Input: part model. Units: mm. Frame: model coordinates. Give positions to 0.01 mm unless a question says otherwise; leave off trailing zeros. Loops run counter-clockwise (first coordinate to the right, second up) from the corner with the lowest first, then second, coordinate; pieces in that order, holes last. Notation, with made-up numbers: M 48,70 L 89,70 A12 cw 89,76 Z; hole C 50,34 d6. An arc over 180 degrees is marked long. Use CSV: the item, a comma, the result in double quotes. Start each with the question number.
Q1. Section A-A, the plane y = -4.25. Output: boundary loops of the cut face in (x, z), plus the area to 3 significant figures.
Q2. Section B-B, the plane z = 21.5. Output: boundary loops of the cut face in (x, y), plus the area to 3 significant figures.
Q3. Material intervals for line 1 along Z through (x, y) = (66, -1); line 2 along X through (y, z) = (-3.5, 13), sorted ascending.
Q4. Section C-C, the plane x = -14. Output: boundary loops of the cut face in (y, z), plus the area to 3 significant figures.
Q5. Pin query (flat end, axial travel): pin 1 (1.9 mm diameter, centred on y = -4.5, z = -3.5, fed in from -X); pin 2 (1.9 mm diameter, centred on x = -59.5, y = -2.5, fed in from -Z); pin 3 (3 mm diameter, centred on y = -4, z = 89, fed in from +X). Return the tip coordinate at first contact, or that it passes through.
from build123d import *

# Parameters (mm, degrees)
F0_W     = 152.4
F0_H     = 101.6
F1_DEPTH = 6.35
F2_W     = 25.4
F2_H     = 6.35
F3_DEPTH = 6.35
F4_W     = 6.35
F4_H     = 25.4
F5_DEPTH = 25.4


with BuildPart() as f1:
    # F0 (on Front) → F1 (new body)
    with BuildSketch(Plane.XZ):
        with Locations((0, 50.8)):
            Rectangle(F0_W, F0_H)
    extrude(amount=F1_DEPTH)

    # F2 (on face) → F3 (join)
    with BuildSketch(Plane.XZ.offset(6.35)):
        with Locations((38.1, -3.175)):
            Rectangle(F2_W, F2_H)
        with Locations((-38.1, -3.175)):
            Rectangle(F2_W, F2_H)
    extrude(amount=-F3_DEPTH)

    # F4 (on face) → F5 (cut)
    with BuildSketch(Plane.XZ.offset(6.35)):
        with Locations((73.025, 88.9)):
            Rectangle(F4_W, F4_H)
        with Locations((73.025, 12.7)):
            Rectangle(F4_W, F4_H)
        with Locations((-73.025, 12.7)):
            Rectangle(F4_W, F4_H)
        with Locations((-73.025, 88.9)):
            Rectangle(F4_W, F4_H)
    extrude(amount=-F5_DEPTH, mode=Mode.SUBTRACT)


solid = f1.part
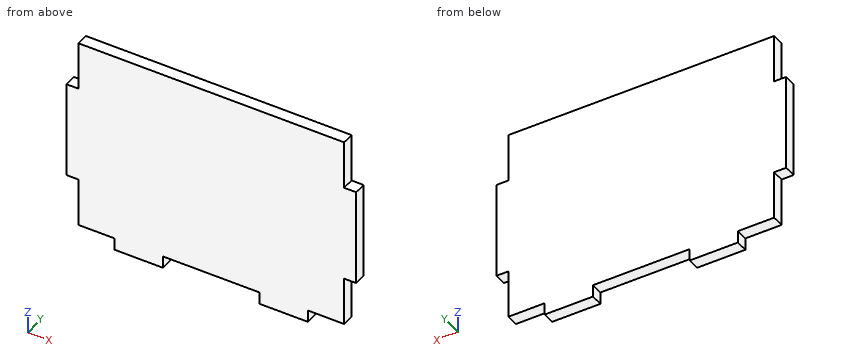
A:
1,outline,"M -76.2,25.4 L -69.85,25.4 L -69.85,0 L -50.8,0 L -50.8,-6.35 L -25.4,-6.35 L -25.4,0 L 25.4,0 L 25.4,-6.35 L 50.8,-6.35 L 50.8,0 L 69.85,0 L 69.85,25.4 L 76.2,25.4 L 76.2,76.2 L 69.85,76.2 L 69.85,101.6 L -69.85,101.6 L -69.85,76.2 L -76.2,76.2 Z"
1,area,"15,200 mm^2"
2,outline,"M -69.85,-6.35 L 69.85,-6.35 L 69.85,0 L -69.85,0 Z"
2,area,"887 mm^2"
3,line 1,"0 to 101.6"
3,line 2,"-69.85 to 69.85"
4,outline,"M -6.35,0 L 0,0 L 0,101.6 L -6.35,101.6 Z"
4,area,"645 mm^2"
5,pin 1,"x = -50.8"
5,pin 2,"z = 0"
5,pin 3,"x = 69.85"
